from build123d import *

# Parameters (mm, degrees)
F1_DEPTH        = 20
F2_R            = 2
F3_R            = 3
F4_R            = 2
F5_W            = 20
F5_H            = 4
F6_DEPTH        = 8.3
F7_R            = 1.6899494937
F9_DEPTH        = 27.6
F12_R           = 4.75
F13_DEPTH       = 10
F15_DEPTH       = 7.6
F17_DEPTH       = 7.6
F19_DEPTH       = 1.5000002459
F21_DEPTH       = 1.5000002459
F23_DEPTH       = 5
F25_DEPTH       = 5
F27_DEPTH       = 2.4358335286
F28_W           = 65.2
F28_H           = 2.6260968298
F29_DEPTH       = 25.7963873446
F31_D           = 4.5
F31_CSINK_D     = 9
F31_CSINK_ANGLE = 90
F33_DEPTH       = 25
F34_W           = 65.2
F34_H           = 34.5529383048
F35_DEPTH       = 10
F36_R           = 2


with BuildPart() as f1:
    # F0 (on Right) → F1 (new body, symmetric)
    with BuildSketch(Plane.YZ):
        Polygon((15.25, 10.5), (-15.25, 10.5), (-15.25, 9.100000374), (13.850000374, 9.100000374), (13.850000374, -10.5), (15.25, -10.5), align=None)
    extrude(amount=F1_DEPTH, both=True)

    # F2
    f2_edges = [f1.edges().sort_by_distance(p)[0] for p in [
        (0, 13.85, 9.1),
    ]]
    fillet(f2_edges, radius=F2_R)

    # F3
    f3_edges = [f1.edges().sort_by_distance(p)[0] for p in [
        (0, 15.25, 10.5),
    ]]
    fillet(f3_edges, radius=F3_R)

    # F4
    f4_edges = [f1.edges().sort_by_distance(p)[0] for p in [
        (20, 14.55, -10.5),
        (20, -15.25, 9.8),
        (-20, -15.25, 9.8),
    ]]
    fillet(f4_edges, radius=F4_R)

    # F5 (on face) → F6 (cut)
    with BuildSketch(Plane(origin=(0, 15.25, 0), x_dir=(-1, 0, 0), z_dir=(0, 1, 0))):
        with Locations((10, -8.5)):
            Rectangle(F5_W, F5_H)
    extrude(amount=-F6_DEPTH, mode=Mode.SUBTRACT)

    # F7
    f7_edges = [f1.edges().sort_by_distance(p)[0] for p in [
        (-20, 14.55, -6.5),
        (0, 14.55, -10.5),
        (0, 14.55, -6.5),
    ]]
    fillet(f7_edges, radius=F7_R)


with BuildPart() as f9:
    # F8 (on Right) → F9 (new body, symmetric)
    with BuildSketch(Plane.YZ):
        with BuildLine():
            Line((12.7858336568, 9.6320193261), (-14.7858336568, 9.6320193261))
            Line((-14.7858336568, 9.6320193261), (-16.5647212416, 9.6320193261))
            Line((-16.5647212416, 9.6320193261), (-16.5647212416, -14.6643677726))
            Line((-16.5647212416, -14.6643677726), (14.7858336568, -14.6643677726))
            Line((14.7858336568, -14.6643677726), (14.7858336568, -9.6320193261))
            Line((14.7858336568, -9.6320193261), (14.7858336568, 7.6320193261))
            ThreePointArc((14.7858336568, 7.6320193261), (14.2000472192, 9.0462328885), (12.7858336568, 9.6320193261))
        make_face()
    extrude(amount=F9_DEPTH, both=True)

    # F10: cut F1
    add(f1.part, mode=Mode.SUBTRACT)

    # F12 (on face) → F13 (cut)
    with BuildSketch(Plane(origin=(0, 13.850000374, 0), x_dir=(-1, 0, 0), z_dir=(0, 1, 0))):
        with Locations((-12.8287095577, -5.3859017789)):
            Circle(F12_R)
    extrude(amount=-F13_DEPTH, mode=Mode.SUBTRACT)

    # F14 (on face) → F15 (join, through all)
    with BuildSketch(Plane.YZ.offset(27.6)):
        with BuildLine():
            Line((16.2858339027, -14.6643677726), (16.2858339027, 7.6320193261))
            ThreePointArc((16.2858339027, 7.6320193261), (15.2607075648, 10.1068932341), (12.7858336568, 11.132019572))
            Line((12.7858336568, 11.132019572), (-16.5647212416, 11.132019572))
            Line((-16.5647212416, 11.132019572), (-16.5647212416, -14.6643677726))
            Line((-16.5647212416, -14.6643677726), (16.2858339027, -14.6643677726))
        make_face()
    extrude(amount=-F15_DEPTH)

    # F16 (on face) → F17 (join, through all)
    with BuildSketch(Plane(origin=(-27.6, 0, 0), x_dir=(0, -1, 0), z_dir=(-1, 0, 0))):
        with BuildLine():
            ThreePointArc((-12.7858336568, 11.132019572), (-15.2607075648, 10.1068932341), (-16.2858339027, 7.6320193261))
            Line((-16.2858339027, 7.6320193261), (-16.2858339027, -14.6643677726))
            Line((-16.2858339027, -14.6643677726), (16.5647212416, -14.6643677726))
            Line((16.5647212416, -14.6643677726), (16.5647212416, 11.132019572))
            Line((16.5647212416, 11.132019572), (-12.7858336568, 11.132019572))
        make_face()
    extrude(amount=-F17_DEPTH)

    # F18 (on face) → F19 (join, through all)
    with BuildSketch(Plane.XY.offset(9.6320193261)):
        with BuildLine():
            Line((-20, -16.5647212416), (20, -16.5647212416))
            Line((20, -16.5647212416), (20, -13.25))
            ThreePointArc((20, -13.25), (19.4142135624, -14.6642135624), (18, -15.25))
            Line((18, -15.25), (-18, -15.25))
            ThreePointArc((-18, -15.25), (-19.4142135624, -14.6642135624), (-20, -13.25))
            Line((-20, -13.25), (-20, -16.5647212416))
        make_face()
    extrude(amount=F19_DEPTH)

    # F20 (on face) → F21 (join, through all)
    with BuildSketch(Plane(origin=(0, 14.7858336568, 0), x_dir=(-1, 0, 0), z_dir=(0, 1, 0))):
        with BuildLine():
            Line((-20, -8.5), (-20, -14.6643677726))
            Line((-20, -14.6643677726), (20, -14.6643677726))
            Line((20, -14.6643677726), (20, -4.8100505063))
            ThreePointArc((20, -4.8100505063), (19.5050252532, -6.0050252532), (18.3100505063, -6.5))
            Line((18.3100505063, -6.5), (1.6899494937, -6.5))
            ThreePointArc((1.6899494937, -6.5), (0.4949747468, -6.9949747468), (0, -8.1899494937))
            Line((0, -8.1899494937), (0, -8.8100505063))
            ThreePointArc((0, -8.8100505063), (-0.4949747468, -10.0050252532), (-1.6899494937, -10.5))
            Line((-1.6899494937, -10.5), (-18, -10.5))
            ThreePointArc((-18, -10.5), (-19.4142135624, -9.9142135624), (-20, -8.5))
        make_face()
    extrude(amount=F21_DEPTH)

    # F22 (on face) → F23 (join)
    with BuildSketch(Plane(origin=(-27.6, 0, 0), x_dir=(0, -1, 0), z_dir=(-1, 0, 0))):
        with BuildLine():
            Line((-16.2858339027, -14.6643677726), (16.5647212416, -14.6643677726))
            Line((16.5647212416, -14.6643677726), (16.5647212416, 11.132019572))
            Line((16.5647212416, 11.132019572), (-12.7858339027, 11.132019572))
            ThreePointArc((-12.7858339027, 11.132019572), (-15.2607076368, 10.1068933061), (-16.2858339027, 7.632019572))
            Line((-16.2858339027, 7.632019572), (-16.2858339027, -14.6643677726))
        make_face()
    extrude(amount=F23_DEPTH)

    # F24 (on face) → F25 (join)
    with BuildSketch(Plane.YZ.offset(27.6)):
        with BuildLine():
            Line((-16.5647212416, 11.132019572), (-16.5647212416, -14.6643677726))
            Line((-16.5647212416, -14.6643677726), (16.2858339027, -14.6643677726))
            Line((16.2858339027, -14.6643677726), (16.2858339027, 7.632019572))
            ThreePointArc((16.2858339027, 7.632019572), (15.2607076368, 10.1068933061), (12.7858339027, 11.132019572))
            Line((12.7858339027, 11.132019572), (-16.5647212416, 11.132019572))
        make_face()
    extrude(amount=F25_DEPTH)

    # F26 (on face) → F27 (cut, through all)
    with BuildSketch(Plane(origin=(0, 16.2858339027, 0), x_dir=(-1, 0, 0), z_dir=(0, 1, 0))):
        with BuildLine():
            Line((1.7086403866, -9.5), (1.7086403866, -8.1106565775))
            Line((1.7086403866, -8.1106565775), (1.7086403866, -7.4905555649))
            ThreePointArc((1.7086403866, -7.4905555649), (1.9546138952, -6.8337115572), (2.5715284873, -6.5))
            Line((2.5715284873, -6.5), (-1.6899494937, -6.5))
            Line((-1.6899494937, -6.5), (-1.6899494937, -10.5))
            Line((-1.6899494937, -10.5), (0.7086403866, -10.5))
            ThreePointArc((0.7086403866, -10.5), (1.4157471677, -10.2071067812), (1.7086403866, -9.5))
        make_face()
        with BuildLine():
            ThreePointArc((2.8457522858, -6.5), (2.7086403866, -6.4905555649), (2.5715284873, -6.5))
            Line((2.5715284873, -6.5), (2.8457522858, -6.5))
        make_face()
    extrude(amount=-F27_DEPTH, mode=Mode.SUBTRACT)

    # F28 (on face) → F29 (join, through all)
    with BuildSketch(Plane.XY.offset(11.132019572)):
        with Locations((0, -17.8777696565)):
            Rectangle(F28_W, F28_H)
    extrude(amount=-F29_DEPTH)

    # F31 (through all)
    with Locations(Plane.XY.offset(11.132019572)):
        with Locations((26.3, -3.2024922073), (-26.3, -3.2024922073)):
            CounterSinkHole(F31_D / 2, F31_CSINK_D / 2, counter_sink_angle=F31_CSINK_ANGLE)

    # F32 (on face) → F33 (cut)
    with BuildSketch(Plane.XY.offset(9.100000374)):
        Polygon((-13.7790497392, -0.699999813), (-13.7790497392, -7.9947467893), (13.7790497392, -7.9947467893), (13.7790497392, 7.9947467893), (-13.7790497392, 7.9947467893), align=None)
    extrude(amount=-F33_DEPTH, mode=Mode.SUBTRACT)

    # F34 (on face) → F35 (join)
    with BuildSketch(Plane.XZ.offset(19.1908180714)):
        with Locations((0, 2.6121013798)):
            Rectangle(F34_W, F34_H)
    extrude(amount=F35_DEPTH)

    # F36
    f36_edges = [f9.edges().sort_by_distance(p)[0] for p in [
        (32.6, -24.190818, 19.888571),
        (-32.6, -24.190818, 19.888571),
        (0, -19.190818, 19.888571),
        (0, -29.190818, 19.888571),
    ]]
    fillet(f36_edges, radius=F36_R)


solid = f9.part
Geometry: final body of the model. Coordinates: model frame, mm. A direction names the side the tool comes from. Give positions to 0.01 mm unless a question says otherwise; leave off trailing zeros. Write each loop counter-clockwise with the first axis right and the second up, starting at its lowest first coordinate (ties: lowest second). Pieces come first, ordered by that corner, then holes. Notation, with made-up numbers: (82, 24) -> (107, 24) arc R20 ccw to (107, 39) -> close; hole circle Ø3 at (-16, 61). An arc over 180 degrees is marked (long way). Answer as a JSON object with one key per item and string values.
1. Contact query for flat-ended pins moving along their axis: pin 1 (1 mm diameter, centred on x = 2.5, z = 10, fed in from +Y); pin 2 (2 mm diameter, centred on x = 23, y = 8.5, fed in from +Z); pin 3 (1.1 mm diameter, centred on x = 16.5, z = -7.5, fed in from +Y). Output: stop coordinate, or through.
Ans:
{"pin 1": "stops at y = -15.25", "pin 2": "stops at z = 11.13", "pin 3": "stops at y = 13.85"}
2. Cut plane C-C on x = -17. Output: boundary loops of the cut face in (y, z), and give its area (3 significant figures).
Ans:
{"outline": "(-29.19, -14.66) -> (16.29, -14.66) -> (16.29, -6.5) -> (13.85, -6.5) -> (13.85, 7.1) arc R2 ccw to (11.85, 9.1) -> (-15.25, 9.1) -> (-15.25, 11.13) -> (-19.19, 11.13) -> (-19.19, 17.89) arc R2 ccw to (-21.19, 19.89) -> (-27.19, 19.89) arc R2 ccw to (-29.19, 17.89) -> close", "area": "1,160 mm^2"}
3. Mould query, pull axis Y, two halves, no side actions, for faces 1 (the flat face through (0, 13.85, 0)), 2 (the flat face through (0, 7.995, -3)), 3 (the flat face through (9, 15, -10.5)). Classes: pulls with the +Y half, pulls with the -Y half, needs draft (parallel to the pull), parting line crosses it, or undercut.
Ans:
{"face 1": "pulls with the +Y half", "face 2": "undercut", "face 3": "needs draft"}
4. Cut plane D-D on y = -9. Output: boundary loops of the cut face in (x, z), and give its area (3 significant figures).
Ans:
{"outline": "(-32.6, -14.66) -> (32.6, -14.66) -> (32.6, 11.13) -> (20, 11.13) -> (20, 9.1) -> (-20, 9.1) -> (-20, 11.13) -> (-32.6, 11.13) -> close", "area": "1,600 mm^2"}
5. Cut plane B-B on z = -4. Output: boundary loops of the cut face in (x, y).
Ans:
{"outline": "(-32.6, -29.19) -> (32.6, -29.19) -> (32.6, 16.29) -> (20, 16.29) -> (20, 13.85) -> (17.37, 13.85) -> (17.37, 3.85) -> (13.78, 3.85) -> (13.78, -7.99) -> (-13.78, -7.99) -> (-13.78, 7.99) -> (8.29, 7.99) -> (8.29, 13.85) -> (-20, 13.85) -> (-20, 16.29) -> (-32.6, 16.29) -> close; hole circle Ø4.5 at (-26.3, -3.2); hole circle Ø4.5 at (26.3, -3.2)"}
6. Cut plane A-A on x = -10. Output: boundary loops of the cut face in (y, z).
Ans:
{"outline": "(-29.19, -14.66) -> (-7.99, -14.66) -> (-7.99, 9.1) -> (-15.25, 9.1) -> (-15.25, 11.13) -> (-19.19, 11.13) -> (-19.19, 17.89) arc R2 ccw to (-21.19, 19.89) -> (-27.19, 19.89) arc R2 ccw to (-29.19, 17.89) -> close; (7.99, -14.66) -> (16.29, -14.66) -> (16.29, -6.5) -> (13.85, -6.5) -> (13.85, 7.1) arc R2 ccw to (11.85, 9.1) -> (7.99, 9.1) -> close"}
7. Ray query, probe 1 along Y at (x, z) = (3, -5.5); probe 2 along Y at (x, z) = (-26.3, -4.5); probe 3 along X at (y, z) = (10, 10.5). Return the intervals inside material, ascending. Write a range as from..to.
Ans:
{"probe 1": "y = -29.19..-7.99, 7.99..13.85", "probe 2": "y = -29.19..-5.45, -0.95..16.29", "probe 3": "x = -32.6..-20, 20..32.6"}
8. Access query for faces 4 (the cylindrical face through (-32.03, -24.261, 19.287)), 5 (the cylindrical face through (17.574, 10.031, -5.177)), 6 (the flat face through (-1.709, 15, -9)), 7 (the flat face through (0, -19.191, 15)). Directions: +Z, -Z, +X, -X, +Y, -Y. A direction counts if a zero-diameter tool reaches every point of the face in a straight line with its end or side. Return the directions, or none.
Ans:
{"face 4": "+Z, -X, +Y, -Y", "face 5": "+Y", "face 6": "+Z, +Y", "face 7": "+Z, +X, -X, +Y"}
